The model under review builds one solid part; all positions refer to its coordinate system, in mm. Face numbers are marked on the shaded views. A direction names the side the tool comes from. Coordinates: 2 decimals unless noted, no trailing zeros. Loops run counter-clockwise (first coordinate to the right, second up) from the corner with the lowest first, then second, coordinate; pieces in that order, holes last. Notation, with made-up numbers: M -14,70 L -8,70 A30 cw -8,104 Z; hole C -27.5,52 d2. An arc over 180 degrees is marked long. Write item = value, one per line. Start each with the question number.
Q1. Wall thickness on probe 1 along Y at (x, z) = (43.5, 36); probe 2 along Z at (x, y) = (-22.5, -40.5); probe 3 along X at (y, z) = (-40, 23.5): over which ranges is each line inside the solid? List them lowest first.
Q2. Clearance check with flat-ended pins moving along their axes: pin 1 Ø1 at (x, z) = (31.5, 4) entering from -Y; pin 2 Ø3 at (x, z) = (-34, 31) entering from +Y. State where each tip first meets the part, or that it passes through.
Q3. Mouldability with a two-part tool opening along Y and no side actions: class the marked faces 3, 4 and 5 as released by +Y, released by -Y, zero draft, split by the parting line, or undercut.
Q4. We need section A-A on y = 0. Give the boundary of the cut face in (x, z), and give its area (4 significant figures).
Q5. For the marked faces 1 and 2, list the 3-axis set-ups (+Z, -Z, +X, -X, +Y, -Y) from which the entire face can be reached by the end or side of a thin tool; tool diameter is ignored.
from build123d import *

# Parameters (mm, degrees)
F0_W     = 98
F0_H     = 98
F1_DEPTH = 38
F2_R     = 20


with BuildPart() as f1:
    # F0 (on Top) → F1 (new body)
    with BuildSketch(Plane.XY):
        Rectangle(F0_W, F0_H)
    extrude(amount=F1_DEPTH)

    # F2
    f2_edges = [f1.edges().sort_by_distance(p)[0] for p in [
        (-49, 49, 19),
        (49, 49, 19),
        (49, -49, 19),
        (-49, -49, 19),
    ]]
    fillet(f2_edges, radius=F2_R)

    # F3 (on Front) → F4 (revolve, cut)
    with BuildSketch(Plane.XZ):
        Polygon((47, 6), (39.5, 0), (54.118488, 0), (54.118488, 6), align=None)
    revolve(axis=Axis((0, 0, 17.541468), (0, 0, -1)), mode=Mode.SUBTRACT)


solid = f1.part
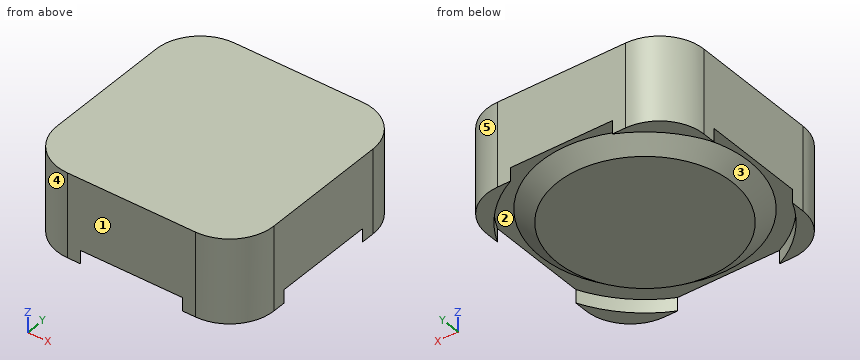
Returned:
q1.probe_1 = -42.77 to 42.77
q1.probe_2 = 5.46 to 38
q1.probe_3 = -45.7 to 45.7
q2.pin_1 = -48.9
q2.pin_2 = 48.69
q3.face_3 = undercut
q3.face_4 = released by -Y
q3.face_5 = released by +Y
q4.outline = M -49,6 L -47,6 L -39.5,0 L 39.5,0 L 47,6 L 49,6 L 49,38 L -49,38 Z
q4.area = 3,655 mm^2
q5.face_1 = +Z, -Z, +X, -X, -Y
q5.face_2 = -Z
